Work out the finished part from the listing and answer in its coordinate system (mm). A direction names the side the tool comes from. Coordinates: 2 decimals unless noted, no trailing zeros. Order: outer loops, then holes, each group sorted by start corner. A loop starts at its lowest first (then second) coordinate and runs counter-clockwise, first axis right, second up. Notation, with made-up numbers: (58.25, 19.5) - (95.25, 19.5) arc R33 cw to (95.25, 52.5) - close; hole circle Ø9 at (-38.5, 42.25). An arc over 180 degrees is marked (long way). Answer as a JSON object with one key per item and string values. Group by question number.
1) Section C-C (x = 10) is taken. Give the vertices of the cut face in (y, z).
2) Section D-D (y = 1.5) is taken. Give the vertices of the cut face in (x, z), plus the area to 3 significant figures.
3) The mould has two halves that part along Y. Classify faces 3 (the face through (11.062, 2.56, 16.87)), 4 (the face through (15, 3, 10)), 5 (the face through (5.7, 0, 9.9)): released by +Y, released by -Y, zero draft, split by the parting line, or undercut.
4) Section B-B (z = 10) is taken. Give the vertices of the cut face in (x, y).
5) Section A-A (y = 3) is taken. Give the vertices of the cut face in (x, z), plus the area to 3 significant figures.
6) A tool of negligible diameter and unlimited length cuts with its end or side. For faces 1 (the face through (7, 3, 20)), 2 (the face through (3.041, 2.56, 11.062)), from which of +Z, -Z, +X, -X, +Y, -Y can it reach the whole face along a straight path? Write none if from no direction.
7) Find the intervals of material crossed by line 1 along Y through (x, z) = (10, 18.25); line 2 along X through (y, z) = (3, 15.75); line 3 along X through (y, z) = (4, 1.5), in increasing order.
8) This flat-tipped pin is pushed along its axis until it touches: P1, Ø1.8, axis at x = 10, y = 3, coming from the -Z side. Where does it stop, or does it pass through?
from build123d import *

# Parameters (mm, degrees)
SKETCH1_W           = 15
SKETCH1_H           = 6
SKETCH1_R           = 1.15
BOSS_EXTRUDE1_DEPTH = 20
SKETCH2_R           = 4
CUT_EXTRUDE2_DEPTH  = 20
CUT_EXTRUDE3_REACH  = 17
SKETCH4_R           = 1.15


with BuildPart() as part:
    # Sketch1 → Boss-Extrude1 (new body)
    with BuildSketch(Plane.XY):
        with Locations((7.5, 3)):
            Rectangle(SKETCH1_W, SKETCH1_H)
        with Locations((10, 3)):
            Circle(SKETCH1_R, mode=Mode.SUBTRACT)
    extrude(amount=BOSS_EXTRUDE1_DEPTH)

    # Sketch2 → Cut-Extrude2 (cut)
    with BuildSketch(Plane.XZ):
        with Locations((10, 10)):
            Circle(SKETCH2_R)
    extrude(amount=-CUT_EXTRUDE2_DEPTH, mode=Mode.SUBTRACT)

    # Sketch4 → Cut-Extrude3 (cut, up to next)
    with BuildSketch(Plane.ZY, mode=Mode.PRIVATE) as cut_extrude3_sk1:
        with Locations((10, 3)):
            Circle(SKETCH4_R)
    cut_extrude3_tool1 = extrude(cut_extrude3_sk1.sketch, amount=-CUT_EXTRUDE3_REACH, mode=Mode.PRIVATE) & part.part
    add(cut_extrude3_tool1.solids().sort_by_distance((0, 3, 10))[0], mode=Mode.SUBTRACT)


solid = part.part
Report:
{
 "1": {"outline": "(0, 0) - (1.85, 0) - (1.85, 6) - (0, 6) - close; (0, 14) - (1.85, 14) - (1.85, 20) - (0, 20) - close; (4.15, 0) - (6, 0) - (6, 6) - (4.15, 6) - close; (4.15, 14) - (6, 14) - (6, 20) - (4.15, 20) - close"},
 "2": {"outline": "(0, 0) - (15, 0) - (15, 20) - (0, 20) - close; hole circle Ø8 at (10, 10)", "area": "250 mm²"},
 "3": {"face 3": "undercut", "face 4": "zero draft", "face 5": "released by -Y"},
 "4": {"outline": "(0, 0) - (6, 0) - (6, 1.85) - (0, 1.85) - close; (0, 4.15) - (6, 4.15) - (6, 6) - (0, 6) - close; (14, 0) - (15, 0) - (15, 6) - (14, 6) - close"},
 "5": {"outline": "(0, 0) - (8.85, 0) - (8.85, 6.17) arc R4 cw to (6.17, 8.85) - (0, 8.85) - close; (0, 11.15) - (6.17, 11.15) arc R4 cw to (8.85, 13.83) - (8.85, 20) - (0, 20) - close; (11.15, 0) - (15, 0) - (15, 20) - (11.15, 20) - (11.15, 13.83) arc R4 cw to (11.15, 6.17) - close", "area": "208 mm²"},
 "6": {"face 1": "+Z, +X, -X, +Y, -Y", "face 2": "-X"},
 "7": {"line 1": "y = 0 to 1.85, 4.15 to 6", "line 2": "x = 0 to 8.85, 11.15 to 15", "line 3": "x = 0 to 9.43, 10.57 to 15"},
 "8": {"P1": "passes through"}
}
